Can you work these out from the model? Positions are in its coordinate system, mm. A direction names the side the tool comes from. Coordinates: 2 decimals unless noted, no trailing zeros. Order: outer loops, then holes, each group sorted by start corner. A loop starts at its lowest first (then second) coordinate and runs counter-clockwise, first axis right, second up. Notation, with made-up numbers: (-20.75, 12) -> (-3.75, 12) arc R17 cw to (-3.75, 18) -> close; hole circle Ø3 at (82.5, 43). An arc over 180 degrees is marked (long way). Return JSON: item names as keys, results as strings. Group by question number.
1) If I drill on probe 1 along X at (y, z) = (1.5, 13.9); probe 2 along X at (y, z) = (4.85, 0); probe 3 along Y at (x, z) = (4, 6), over which ranges is the centre line in solid material (lowest first)? Write a range as from..to.
2) If we section it at D-D, the plane z = -7.5: Please give me the cut outline in (x, y).
3) For faces 1 (the flat face through (0, 0, 19)), 2 (the cylindrical face through (-9, 4, 0)), 3 (the flat face through (5, -3, 17)), 4 (the flat face through (0, 4, -8)), which set-ups out of +Z, -Z, +X, -X, +Y, -Y let a thin tool reach every point of the face, with its end or its side?
4) For pin 1 (2 mm diameter, centred on x = 3, y = 3.5, fed in from -Z); pin 2 (3 mm diameter, centred on x = 12.5, z = 15.5, fed in from +Y); pin 3 (1.5 mm diameter, centred on x = -3, z = 3.5, fed in from -Y); pin 4 (1.6 mm diameter, centred on x = -13.9, z = -13.9, fed in from -Y), each with a flat end and sliding along its axis, tell me the tip position at first contact or that it passes through.
5) Thinking about a two-plate mould opening in X: for faces 5 (the flat face through (-10, 2, 0)), 6 (the flat face through (6, 9, -2)), 7 (the cylindrical face through (-12, 4, 0)), 8 (the cylindrical face through (-7.81, 14.46, -1.73)), which applies, +X half, -X half, draft (parallel to the pull), parting line (faces both ways), or undercut?
6) If we section it at A-A, the plane x = 13.9: Please give me the cut outline in (y, z).
7) If we section it at B-B, the plane z = 13.9: Please give me the cut outline in (x, y), then the cut area to 3 significant figures.
8) If we section it at C-C, the plane y = 1.5: Please give me the cut outline in (x, z).
from build123d import *

# Parameters (mm, degrees)
SKETCH1_W           = 32
SKETCH1_H           = 32
SKETCH1_R           = 1
BOSS_EXTRUDE1_DEPTH = 2
SKETCH2_R           = 1
BOSS_EXTRUDE2_DEPTH = 4
SKETCH3_R           = 8
BOSS_EXTRUDE3_DEPTH = 3
SKETCH4_R           = 6
BOSS_EXTRUDE4_DEPTH = 3
SKETCH5_R           = 8
BOSS_EXTRUDE5_DEPTH = 5
SKETCH_1_W          = 10
SKETCH_1_H          = 4.5
EXTRUDE_1_DEPTH     = 7
SKETCH_2_W          = 10
SKETCH_2_H          = 5
EXTRUDE_2_DEPTH     = 6


with BuildPart() as part:
    # Sketch1 → Boss-Extrude1 (new body)
    with BuildSketch(Plane(origin=(0, 0, 0), x_dir=(1, 0, 0), z_dir=(0, 1, 0))):
        Rectangle(SKETCH1_W, SKETCH1_H)
        with Locations(Location((-13.9, 13.9, 0), (0, 0, 270))):
            Circle(SKETCH1_R, mode=Mode.SUBTRACT)
        with Locations(Location((13.9, 13.9, 0), (0, 0, 270))):
            Circle(SKETCH1_R, mode=Mode.SUBTRACT)
        with Locations(Location((-13.9, -13.9, 0), (0, 0, 270))):
            Circle(SKETCH1_R, mode=Mode.SUBTRACT)
        with Locations(Location((13.9, -13.9, 0), (0, 0, 270))):
            Circle(SKETCH1_R, mode=Mode.SUBTRACT)
    extrude(amount=BOSS_EXTRUDE1_DEPTH)

    # Sketch2 → Boss-Extrude2 (add)
    with BuildSketch(Plane(origin=(0, 2, 0), x_dir=(1, 0, 0), z_dir=(0, 1, 0))):
        with BuildLine():
            Line((-8, -8), (8, -8))
            Line((8, -8), (8, -2))
            Line((8, -2), (10, -2))
            ThreePointArc((10, -2), (12, 0), (10, 2))
            Line((10, 2), (8, 2))
            Line((8, 2), (8, 8))
            Line((8, 8), (-8, 8))
            Line((-8, 8), (-8, 2))
            Line((-8, 2), (-10, 2))
            ThreePointArc((-10, 2), (-12, 0), (-10, -2))
            Line((-10, -2), (-8, -2))
            Line((-8, -2), (-8, -8))
        make_face()
        with Locations(Location((10, 0, 0), (0, 0, 270))):
            Circle(SKETCH2_R, mode=Mode.SUBTRACT)
        with Locations(Location((-10, 0, 0), (0, 0, 270))):
            Circle(SKETCH2_R, mode=Mode.SUBTRACT)
    extrude(amount=BOSS_EXTRUDE2_DEPTH)

    # Sketch3 → Boss-Extrude3 (add)
    with BuildSketch(Plane(origin=(0, 6, 0), x_dir=(1, 0, 0), z_dir=(0, 1, 0))):
        with Locations(Location((0, 0, 0), (0, 0, 270))):
            Circle(SKETCH3_R)
    extrude(amount=BOSS_EXTRUDE3_DEPTH)

    # Sketch4 → Boss-Extrude4 (add)
    with BuildSketch(Plane(origin=(0, 9, 0), x_dir=(1, 0, 0), z_dir=(0, 1, 0))):
        with Locations(Location((0, 0, 0), (0, 0, 270))):
            Circle(SKETCH4_R)
    extrude(amount=BOSS_EXTRUDE4_DEPTH)

    # Sketch5 → Boss-Extrude5 (add)
    with BuildSketch(Plane(origin=(0, 12, 0), x_dir=(1, 0, 0), z_dir=(0, 1, 0))):
        with Locations(Location((0, 0, 0), (0, 0, 270))):
            Circle(SKETCH5_R)
    extrude(amount=BOSS_EXTRUDE5_DEPTH)

    # 草图1 → 凸台-拉伸1 (add)
    with BuildSketch(Plane.XZ):
        with Locations((0, 13.9)):
            Rectangle(SKETCH_1_W, SKETCH_1_H)
    extrude(amount=EXTRUDE_1_DEPTH)

    # 草图2 → 凸台-拉伸2 (add)
    with BuildSketch(Plane.XY.offset(16.15)):
        with Locations((0, -2.5)):
            Rectangle(SKETCH_2_W, SKETCH_2_H)
    extrude(amount=EXTRUDE_2_DEPTH)


solid = part.part
Result sheet:
{
 "1": {"probe 1": "x = -16..-14.9, -12.9..12.9, 14.9..16", "probe 2": "x = -12..-11, -9..9, 11..12", "probe 3": "y = 0..9, 12..17"},
 "2": {"outline": "(-16, 0) -> (16, 0) -> (16, 2) -> (8, 2) -> (8, 6) -> (2.78, 6) -> (2.78, 9) -> (-2.78, 9) -> (-2.78, 6) -> (-8, 6) -> (-8, 2) -> (-16, 2) -> close; (-2.78, 12) -> (2.78, 12) -> (2.78, 17) -> (-2.78, 17) -> close"},
 "3": {"face 1": "+Z, +X, -X, +Y", "face 2": "+Y", "face 3": "+Z, -Z, +X, -Y", "face 4": "-Z, +X, -X, +Y"},
 "4": {"pin 1": "stops at z = -8", "pin 2": "stops at y = 2", "pin 3": "stops at y = 0", "pin 4": "passes through"},
 "5": {"face 5": "undercut", "face 6": "draft", "face 7": "-X half", "face 8": "parting line"},
 "6": {"outline": "(0, -16) -> (2, -16) -> (2, -14.9) -> (0, -14.9) -> close; (0, -12.9) -> (2, -12.9) -> (2, 12.9) -> (0, 12.9) -> close; (0, 14.9) -> (2, 14.9) -> (2, 16) -> (0, 16) -> close"},
 "7": {"outline": "(-16, 0) -> (-14.9, 0) -> (-14.9, 2) -> (-16, 2) -> close; (-12.9, 0) -> (-5, 0) -> (-5, -7) -> (5, -7) -> (5, 0) -> (12.9, 0) -> (12.9, 2) -> (-12.9, 2) -> close; (14.9, 0) -> (16, 0) -> (16, 2) -> (14.9, 2) -> close", "area": "126 mm2"},
 "8": {"outline": "(-16, -16) -> (16, -16) -> (16, 16) -> (-16, 16) -> close; hole circle Ø2 at (-13.9, -13.9); hole circle Ø2 at (-13.9, 13.9); hole circle Ø2 at (13.9, -13.9); hole circle Ø2 at (13.9, 13.9)"}
}
